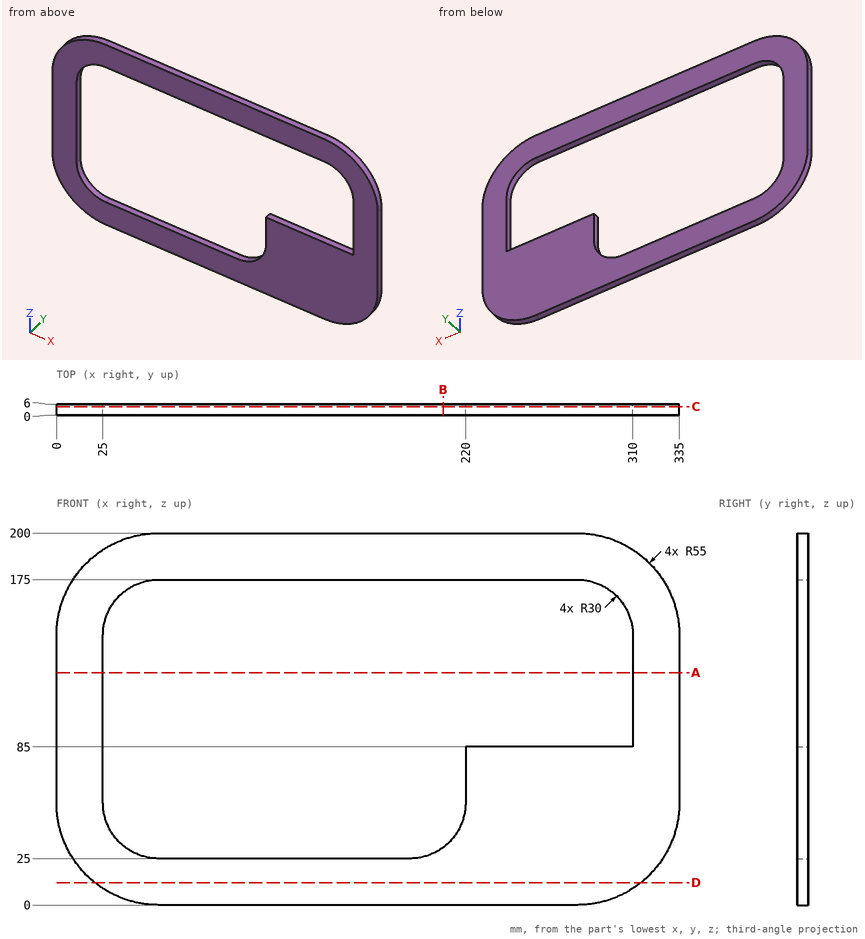
The figure shows three views and two pictorial views of one solid part (mm, origin at its lowest corner). Answer the questions. Give positions to 0.01 mm unless a question says otherwise; leave off trailing zeros. Write each loop counter-clockwise with the first axis right and the second up, starting at its lowest first coordinate (ties: lowest second). Pieces come first, ordered by that corner, then holes. Notation, with made-up numbers: M -5.5,-17.75 L 1.5,-17.75 A14 ccw 1.5,-9.75 Z; hole C 86,65.25 d1. An arc over 180 degrees is marked long. One line per item, written item: value. Start each with the question number.
(1) Find section C-C (y = 4.55). Determine the outline of the cut face in (x, z), plus the area to 3 significant figures.
(2) Find section B-B (x = 208). Determine the outline of the cut face in (y, z).
(3) Flat-ended cylindrical pins translate along their axes: pin 1 Ø12 at (x, z) = (220.5, 37) entering from -Y; pin 2 Ø1.5 at (x, y) = (293, 4) entering from +Z; pin 3 Ø6 at (x, z) = (283.5, 169.5) entering from +Y. Find the tip coordinate at first contact, or state that the pin passes through.
(4) Find section A-A (z = 125). Determine the outline of the cut face in (x, y).
(5) Find section D-D (z = 12). Determine the outline of the cut face in (x, y), plus the area to 3 significant figures.
(6) Find the intervals of material crossed by line 1 (Z direction, x = 92.5, y = 4.7); line 2 (X direction, y = 3.6, z = 71); line 3 (X direction, y = 1.95, z = 136.5), in increasing order.
Results below:
1. outline: M 0,55 A55 ccw 55,0 L 280,0 A55 ccw 335,55 L 335,145 A55 ccw 280,200 L 55,200 A55 ccw 0,145 Z; hole M 25,55 A30 ccw 55,25 L 190,25 A30 ccw 220,55 L 220,85 L 310,85 L 310,145 A30 ccw 280,175 L 55,175 A30 ccw 25,145 Z
1. area: 27,800 mm^2
2. outline: M 0,0 L 6,0 L 6,31 L 0,31 Z; M 0,175 L 6,175 L 6,200 L 0,200 Z
3. pin 1: stops at y = 0
3. pin 2: stops at z = 198.62
3. pin 3: passes through
4. outline: M 0,0 L 25,0 L 25,6 L 0,6 Z; M 310,0 L 335,0 L 335,6 L 310,6 Z
5. outline: M 20.71,0 L 314.29,0 L 314.29,6 L 20.71,6 Z
5. area: 1,760 mm^2
6. line 1: z = 0 to 25, 175 to 200
6. line 2: x = 0 to 25, 220 to 335
6. line 3: x = 0 to 25, 310 to 335
